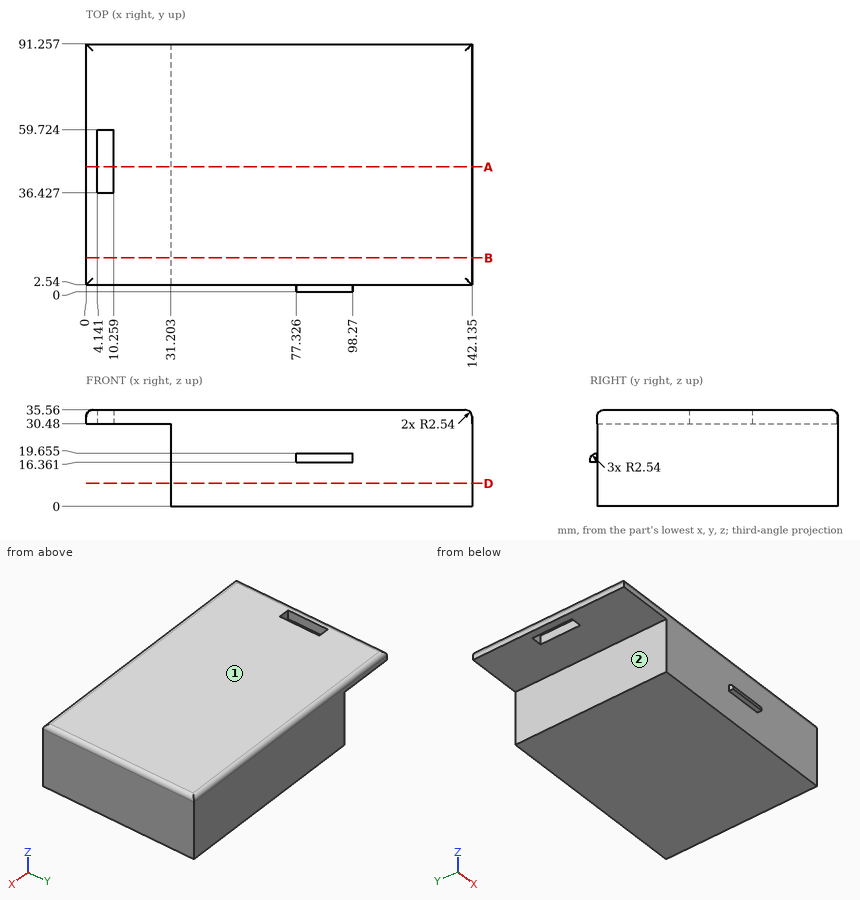
Check sheet for the drawn part. Datum: minimum x, y, z corner. Units: mm. A direction names the side the tool comes from. Coordinates: 2 decimals unless noted, no trailing zeros. Order: outer loops, then holes, each group sorted by start corner. A loop starts at its lowest first (then second) coordinate and runs counter-clockwise, first axis right, second up. Notation, with made-up numbers: (-7, -35.5) - (20, -35.5) arc R21 cw to (20, -14.5) - close; hole circle Ø5 at (-25.5, 23.5). An arc over 180 degrees is marked (long way). Return JSON: item names as keys, results as strings.
(1) Go/stop test with flat-tipped pins: pin 1 (5.5 mm diameter, centred on x = 6.5, z = 32.5, fed in from -Y); pin 2 (1.3 mm diameter, centred on x = 88, y = 1.5, fed in from -Z); pin 3 (15.5 mm diameter, centred on x = 19.5, y = 33, fed in from -Z). Record where each tip stops, or that it passes through.
Filled sheet:
{"pin 1": "stops at y = 2.54", "pin 2": "stops at z = 16.36", "pin 3": "stops at z = 30.48"}
(2) Access from +Z, -Z, +X, -X, +Y, -Y to the whole of each face (thin tool, end or side, straight path). Record for the marked faces 1 and 2.
Filled sheet:
{"face 1": "+Z, +X, -X, +Y, -Y", "face 2": "-Z, -X, +Y, -Y"}
(3) Thickness scan on line 1 along X through (y, z) = (40.5, 2) (1 decimal); line 2 along Y through (x, z) = (129, 10.5); line 3 along X through (y, z) = (51.5, 33.5) (1 decimal). Record the ranges inside material, lowest first.
Filled sheet:
{"line 1": "x = 31.2 to 142.1", "line 2": "y = 2.54 to 91.26", "line 3": "x = 0 to 4.1, 10.3 to 142.1"}
(4) Section check B-B, the plane y = 12.5. Record the cut outline in (x, z) (1 decimal).
Filled sheet:
{"outline": "(0, 30.5) - (31.2, 30.5) - (31.2, 0) - (142.1, 0) - (142.1, 33) arc R2.5 ccw to (139.6, 35.6) - (2.5, 35.6) arc R2.5 ccw to (0, 33) - close"}
(5) Section check D-D, the plane z = 8.5. Record the cut outline in (x, y) (1 decimal), and give its area (3 significant figures).
Filled sheet:
{"outline": "(31.2, 2.5) - (142.1, 2.5) - (142.1, 91.3) - (31.2, 91.3) - close", "area": "9,840 mm^2"}
(6) Section check A-A, the plane y = 46. Record the cut outline in (x, z) (1 decimal), and give its area (3 significant figures).
Filled sheet:
{"outline": "(0, 30.5) - (4.1, 30.5) - (4.1, 35.6) - (2.5, 35.6) arc R2.5 ccw to (0, 33) - close; (10.3, 30.5) - (31.2, 30.5) - (31.2, 0) - (142.1, 0) - (142.1, 33) arc R2.5 ccw to (139.6, 35.6) - (10.3, 35.6) - close", "area": "4,070 mm^2"}
